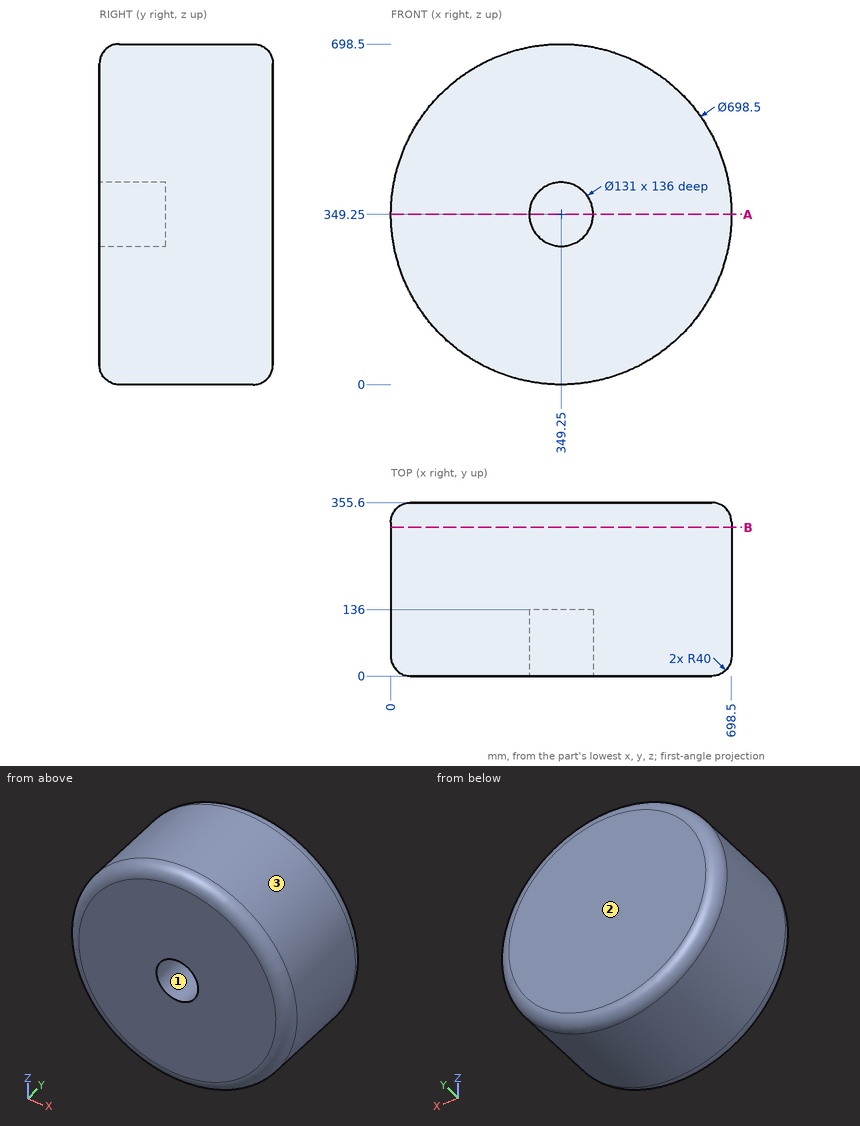
Verification items for this drawing (mm, ordinates from the low corner). Coordinates: 2 decimals unless noted, no trailing zeros. Write each loop counter-clockwise with the first axis right and the second up, starting at its lowest first coordinate (ties: lowest second). Pieces come first, ordered by that corner, then holes. Notation, with made-up numbers: M 84.5,58.5 L 90.5,58.5 A12 ccw 90.5,71.5 Z; hole C 4,36.25 d9. An arc over 180 degrees is marked long. Use one line per item in the form item = value. Start each with the question number.
1) Release check for a two-part mould opening along X. For the marked faces 1, 2 and 3 record: pulls with the +X half, pulls with the -X half, needs draft (parallel to the pull), parting line crosses it, or undercut.
2) Section check B-B on y = 305. Enter the section's corners in (x, z).
3) Section check A-A on z = 349.25. Enter the section's corners in (x, y), and give its area (3 significant figures).
4) Go/stop test with flat-tipped pins: pin 1 Ø12 at (x, y) = (331.5, 38) entering from +Z; pin 2 Ø1 at (x, y) = (604.5, 42.5) entering from -Z; pin 3 Ø4 at (x, y) = (428.5, 126) entering from -Z. Record where each tip stops, or that it passes through.
5) Thickness scan on probe 1 along X at (y, z) = (51, 349.25); probe 2 along Z at (x, y) = (373, 121). Record the ranges inside material, lowest first. Write a range as from..to.
Responses:
q1.face_1 = undercut
q1.face_2 = needs draft
q1.face_3 = parting line crosses it
q2.outline = C 349.25,349.25 d698.5
q3.outline = M 0,40 A40 ccw 40,0 L 283.75,0 L 283.75,136 L 414.75,136 L 414.75,0 L 658.5,0 A40 ccw 698.5,40 L 698.5,315.6 A40 ccw 658.5,355.6 L 40,355.6 A40 ccw 0,315.6 Z
q3.area = 229,000 mm2
q4.pin_1 = 698.29
q4.pin_2 = 110.34
q4.pin_3 = 8.65
q5.probe_1 = 0..283.75, 414.75..698.5
q5.probe_2 = 0.81..288.21, 410.29..697.69
